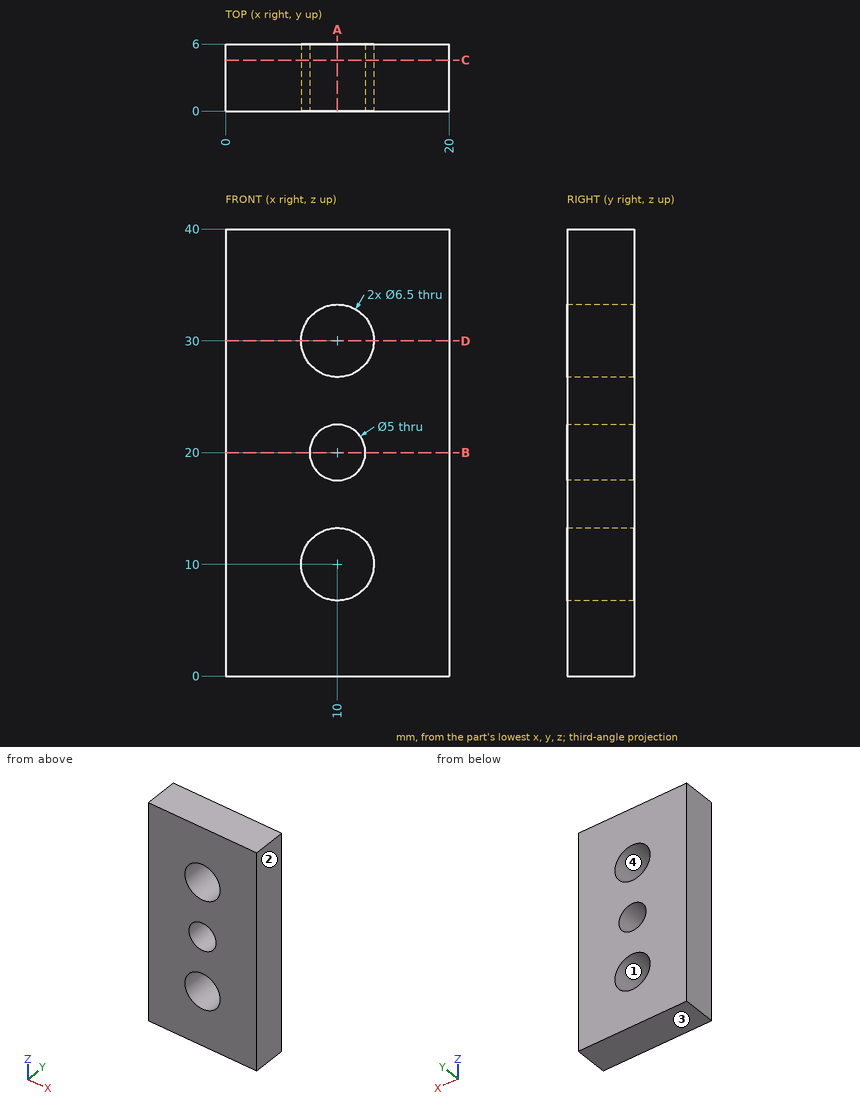
Part print with two shaded views. Sizes in mm from the minimum x, y, z corner. Round coordinates to 2 decimals unless told otherwise and drop trailing zeros. Loops run counter-clockwise (first coordinate to the right, second up) from the corner with the lowest first, then second, coordinate; pieces in that order, holes last.
Item 1: Saw through at C-C (y = 4.55). List the corners of the cut face in (x, z).
Item 2: Saw through at B-B (z = 20). List the corners of the cut face in (x, y).
Item 3: Drill centre lines: line 1 along X through (y, z) = (5.45, 20); line 2 along Z through (x, y) = (7.25, 1.75); line 3 along X through (y, z) = (4.1, 10). Where is each one in solid material? Low to high.
Item 4: Saw through at D-D (z = 30). List the corners of the cut face in (x, y).
Item 5: Saw through at A-A (x = 10). List the corners of the cut face in (y, z), then the cut area to 3 significant figures.
Item 6: Two-plate mould, pull along Z, no slides. Class the marked faces 1, 2, 3 and 4: released by +Z, released by -Z, zero draft, split by the parting line, or undercut.
Item 7: Pin check, flat tip, straight feed: P1, Ø2, axis at x = 7.5, z = 12, coming from the +Y side. Stop position of the tip, or through.
Worked answers:
1. outline: (0, 0) - (20, 0) - (20, 40) - (0, 40) - close; hole circle Ø6.5 at (10, 10); hole circle Ø6.5 at (10, 30); hole circle Ø5 at (10, 20)
2. outline: (0, 0) - (7.5, 0) - (7.5, 6) - (0, 6) - close; (12.5, 0) - (20, 0) - (20, 6) - (12.5, 6) - close
3. line 1: x = 0 to 7.5, 12.5 to 20
3. line 2: z = 0 to 8.27, 11.73 to 28.27, 31.73 to 40
3. line 3: x = 0 to 6.75, 13.25 to 20
4. outline: (0, 0) - (6.75, 0) - (6.75, 6) - (0, 6) - close; (13.25, 0) - (20, 0) - (20, 6) - (13.25, 6) - close
5. outline: (0, 0) - (6, 0) - (6, 6.75) - (0, 6.75) - close; (0, 13.25) - (6, 13.25) - (6, 17.5) - (0, 17.5) - close; (0, 22.5) - (6, 22.5) - (6, 26.75) - (0, 26.75) - close; (0, 33.25) - (6, 33.25) - (6, 40) - (0, 40) - close
5. area: 132 mm2
6. face 1: undercut
6. face 2: zero draft
6. face 3: released by -Z
6. face 4: undercut
7. P1: stops at y = 6
